Part model, mm, in its own coordinate system. A direction names the side the tool comes from. Give positions to 0.01 mm unless a question says otherwise; leave off trailing zeros. Write each loop counter-clockwise with the first axis right and the second up, starting at its lowest first coordinate (ties: lowest second). Pieces come first, ordered by that corner, then holes.
```python
from build123d import *

# Parameters (mm, degrees)
SKETCH1_W                   = 64
SKETCH1_H                   = 62
SKETCH1_R                   = 2.5
SKETCH1_R_2                 = 3
BOSS_EXTRUDE1_DEPTH         = 6
CUT_EXTRUDE2_REACH          = 8
FILLET2_R                   = 3
TAP_DRILL_FOR_M3_TAP1_D     = 2.5
TAP_DRILL_FOR_M3_TAP1_DEPTH = 9
TAP_DRILL_FOR_M3_TAP1_TIP   = 0.751075774
CUT_EXTRUDE3_DEPTH          = 8
CUT_EXTRUDE4_DEPTH          = 3
FILLET3_R                   = 3
CUT_EXTRUDE5_REACH          = 5
SKETCH14_R                  = 1.5
SKETCH15_R                  = 2.5
CUT_EXTRUDE6_DEPTH          = 6
LPATTERN3_COUNT             = 3
LPATTERN3_PITCH             = 4
FILLET4_R                   = 1
SKETCH16_W                  = 22.057961884
SKETCH16_H                  = 6
CUT_EXTRUDE7_DEPTH          = 1


with BuildPart() as part:
    # Sketch1 → Boss-Extrude1 (new body)
    with BuildSketch(Plane(origin=(0, 0, 0), x_dir=(0, 0, -1), z_dir=(1, 0, 0))):
        with Locations((32, 31)):
            Rectangle(SKETCH1_W, SKETCH1_H)
        with Locations((6, 14.5)):
            Circle(SKETCH1_R, mode=Mode.SUBTRACT)
        with Locations((50, 44)):
            Circle(SKETCH1_R_2, mode=Mode.SUBTRACT)
    extrude(amount=BOSS_EXTRUDE1_DEPTH)

    # Sketch3 → Cut-Extrude2 (cut, up to next)
    with BuildSketch(Plane(origin=(6, 0, 0), x_dir=(0, 0, -1), z_dir=(1, 0, 0)), mode=Mode.PRIVATE) as cut_extrude2_sk1:
        Polygon((64, 0), (52, 0), (54.225932994, 25.442530542), (64, 29), align=None)
    cut_extrude2_tool1 = extrude(cut_extrude2_sk1.sketch, amount=-CUT_EXTRUDE2_REACH, mode=Mode.PRIVATE) & part.part
    add(cut_extrude2_tool1.solids().sort_by_distance((6, 13.1347, -58.667711))[0], mode=Mode.SUBTRACT)

    # Fillet2
    fillet2_edges = [part.edges().sort_by_distance(p)[0] for p in [
        (3, 25.442530542, -54.225932994),
    ]]
    fillet(fillet2_edges, radius=FILLET2_R)

    # Tap Drill for M3 Tap1
    with Locations(Plane(origin=(0, 0, 0), x_dir=(-1, 0, 0), z_dir=(0, -1, 0))):
        with Locations((-3, 48), (-3, 12)):
            Hole(TAP_DRILL_FOR_M3_TAP1_D / 2, depth=TAP_DRILL_FOR_M3_TAP1_DEPTH)
            with Locations((0, 0, -(TAP_DRILL_FOR_M3_TAP1_DEPTH + TAP_DRILL_FOR_M3_TAP1_TIP / 2))):  # 118° drill point
                Cone(0, TAP_DRILL_FOR_M3_TAP1_D / 2, TAP_DRILL_FOR_M3_TAP1_TIP, mode=Mode.SUBTRACT)

    # Sketch9 → Cut-Extrude3 (cut)
    with BuildSketch(Plane(origin=(6, 0, 0), x_dir=(0, 0, -1), z_dir=(1, 0, 0))):
        with BuildLine():
            Line((7.718264205, 20.248701429), (27.783442934, 14.251298571))
            ThreePointArc((27.783442934, 14.251298571), (32.652701535, 14.894000165), (35.410553657, 18.958110934))
            Line((35.410553657, 18.958110934), (43, 62))
            Line((43, 62), (0, 62))
            Line((0, 62), (0, 14.5))
            ThreePointArc((0, 14.5), (2.415978881, 19.311942707), (7.718264205, 20.248701429))
        make_face()
    extrude(amount=-CUT_EXTRUDE3_DEPTH, mode=Mode.SUBTRACT)

    # Sketch13 → Cut-Extrude4 (cut)
    with BuildSketch(Plane(origin=(6, 0, 0), x_dir=(0, 0, -1), z_dir=(1, 0, 0))):
        Polygon((54, 35), (64, 35), (64, 62), (43, 62), (37.457598082, 30.567476765), align=None)
    extrude(amount=-CUT_EXTRUDE4_DEPTH, mode=Mode.SUBTRACT)

    # Fillet3
    fillet3_edges = [part.edges().sort_by_distance(p)[0] for p in [
        (1.5, 62, -43),
    ]]
    fillet(fillet3_edges, radius=FILLET3_R)

    # Sketch14 → Cut-Extrude5 (cut, up to next)
    with BuildSketch(Plane(origin=(3, 0, 0), x_dir=(0, 0, -1), z_dir=(1, 0, 0)), mode=Mode.PRIVATE) as cut_extrude5_sk1:
        with Locations((56, 59)):
            Circle(SKETCH14_R)
    cut_extrude5_tool1 = extrude(cut_extrude5_sk1.sketch, amount=-CUT_EXTRUDE5_REACH, mode=Mode.PRIVATE) & part.part
    add(cut_extrude5_tool1.solids().sort_by_distance((3, 59, -56))[0], mode=Mode.SUBTRACT)
    # Sketch14 → Cut-Extrude5 (cut, up to next)
    with BuildSketch(Plane(origin=(3, 0, 0), x_dir=(0, 0, -1), z_dir=(1, 0, 0)), mode=Mode.PRIVATE) as cut_extrude5_sk2:
        with Locations((46, 59)):
            Circle(SKETCH14_R)
    cut_extrude5_tool2 = extrude(cut_extrude5_sk2.sketch, amount=-CUT_EXTRUDE5_REACH, mode=Mode.PRIVATE) & part.part
    add(cut_extrude5_tool2.solids().sort_by_distance((3, 59, -46))[0], mode=Mode.SUBTRACT)

    # Sketch15 → Cut-Extrude6 (cut)
    with BuildSketch(Plane.ZY):
        with Locations((-9.832467619, 13.35449053)):
            Circle(SKETCH15_R)
    cut_extrude6 = extrude(amount=-CUT_EXTRUDE6_DEPTH, mode=Mode.SUBTRACT)

    # LPattern3: Cut-Extrude6 ×3
    with Locations(*[Vector(0, -0.286377368, -0.958116905) * (i * LPATTERN3_PITCH) for i in range(1, LPATTERN3_COUNT)]):
        add(cut_extrude6, mode=Mode.SUBTRACT)

    # Fillet4
    fillet4_edges = [part.edges().sort_by_distance(p)[0] for p in [
        (3, 15.364420622, -8.345799861),
        (3, 12.490069908, -7.486667758),
        (3, 14.218911152, -12.17826748),
        (3, 11.344560437, -11.319135378),
        (3, 10.199050967, -15.151602997),
        (3, 13.073401682, -16.0107351),
    ]]
    fillet(fillet4_edges, radius=FILLET4_R)

    # Sketch16 → Cut-Extrude7 (cut)
    with BuildSketch(Plane(origin=(3, 0, 0), x_dir=(0, 0, -1), z_dir=(1, 0, 0))):
        with Locations((52.971019058, 59)):
            Rectangle(SKETCH16_W, SKETCH16_H)
    extrude(amount=-CUT_EXTRUDE7_DEPTH, mode=Mode.SUBTRACT)


solid = part.part
```
1) Wall check: L1, parallel to X at y = 2.5, z = -12; L2, parallel to Y at x = 1.05, z = -46; L3, parallel to Y at x = 0.65, z = -56. Give the ranges that are in metal, low to high.
Answers follow:
L1: x = 0 to 1.75, 4.25 to 6
L2: y = 0 to 57.5, 60.5 to 62
L3: y = 26.09 to 57.5, 60.5 to 62
2) Two-plate mould, pull along Y, no slides. Class faces 6 (the face through (3, 0, -26)), 7 (the face through (1.014, 60.265, -56.806)), 8 (the face through (0, 25, -39)), 9 (the face through (4.52, 32.75, -45.61)): +Y half, -Y half, draft (parallel to the pull), parting line (faces both ways), or undercut.
Answers follow:
face 6: -Y half
face 7: undercut
face 8: draft
face 9: +Y half
3) Pin check, flat tips, straight feed: pin 1 Ø5 at (y, z) = (59, -53) entering from +X; pin 2 Ø3.5 at (y, z) = (59, -56) entering from -X; pin 3 Ø3 at (x, z) = (3, -12) entering from +Y; pin 4 Ø1.5 at (x, y) = (1.5, 44) entering from +Z. Stop position of each tip, or through.
Answers follow:
pin 1: stops at x = 2
pin 2: stops at x = 0
pin 3: stops at y = 19.42
pin 4: stops at z = -39.69
4) Saw through at B-B, the plane y = 32.5. Write the cut outline in (x, z), then the cut area to 3 significant figures.
Answers follow:
outline: (0, -64) - (6, -64) - (6, -44.67) - (3, -44.67) - (3, -37.8) - (0, -37.8) - close
area: 137 mm2
5) Saw through at A-A, the plane z = -50. Write the cut outline in (x, y), then the cut area to 3 significant figures.
Answers follow:
outline: (0, 0) - (6, 0) - (6, 33.93) - (3, 33.93) - (3, 41) - (0, 41) - close; (0, 47) - (3, 47) - (3, 56) - (2, 56) - (2, 62) - (0, 62) - close
area: 264 mm2
6) 3-axis set-ups, long thin cutter, end or side, ignore diameter. For faces 1 (the face through (3, 43, -53)), 2 (the face through (2.958, 15.756, -10.528)), 3 (the face through (3.042, 17.292, -17.61)), 4 (the face through (2, 59, -53)), 5 (the face through (2.84, 4.56, -49.24)): which of +Z, -Z, +X, -X, +Y, -Y reach the whole face in a straight line?
Answers follow:
face 1: +Z, +X, +Y
face 2: +X, -X
face 3: +X, -X, +Y
face 4: +Z, -Z, +X, +Y
face 5: -Y
